Input: part model. Units: mm. Frame: model coordinates. Face numbers are marked on the shaded views. Coordinates: 2 decimals unless noted, no trailing zeros. Loops run counter-clockwise (first coordinate to the right, second up) from the corner with the lowest first, then second, coordinate; pieces in that order, holes last.
Item 1: Ray query, line 1 along Z through (x, y) = (0, 2.2); line 2 along X through (y, z) = (1.1, 0); line 3 along Z through (x, y) = (-5.5, 4.6). Return the intervals inside material, ascending.
Item 2: Pull-direction query (X, two-part tool) for the marked faces 1, 2 and 3; classes: released by +X, released by -X, zero draft, split by the parting line, or undercut.
Item 3: Contact query for flat-ended pins moving along their axis: P1, Ø6, axis at x = 4, z = 1.5, coming from the -Y side; P2, Ø2, axis at y = 2.5, z = 5.5, coming from the +X side; P3, Ø1.5, axis at x = 0, z = 0, coming from the -Y side. Output: stop coordinate, or through.
Item 4: Section B-B on x = -9.5. Return loops of the section in (y, z).
Item 5: Section C-C on z = -8. Return loops of the section in (x, y), and give its area (3 significant figures).
```python
from build123d import *

# Parameters (mm, degrees)
SKETCH1_R           = 1.218989221
BOSS_EXTRUDE6_DEPTH = 5.08


with BuildPart() as part:
    # Sketch1 → Boss-Extrude6 (new body)
    with BuildSketch(Plane(origin=(0, 0, 0), x_dir=(1, 0, 0), z_dir=(0, 1, 0))):
        with BuildLine():
            ThreePointArc((-1.519001557, -12.033660962), (0, -12.662852008), (1.519001557, -12.033660962))
            Line((1.519001557, -12.033660962), (2.038136122, -11.193432272))
            ThreePointArc((2.038136122, -11.193432272), (2.034563062, -11.204068286), (2.030934498, -11.214685493))
            Line((2.030934498, -11.214685493), (10.329167319, 2.060586649))
            ThreePointArc((10.329167319, 2.060586649), (7.892426257, 9.808202336), (-0.164422722, 8.783292397))
            ThreePointArc((-0.164422722, 8.783292397), (-8.079308366, 9.623050723), (-10.561191909, 2.060586649))
            Line((-10.561191909, 2.060586649), (-9.239218773, 0))
            Line((-9.239218773, 0), (-9.150338425, -0.138539621))
            Line((-9.150338425, -0.138539621), (-2.013925132, -11.262213432))
            Line((-2.013925132, -11.262213432), (-1.519001557, -12.033660962))
        make_face()
        Circle(SKETCH1_R, mode=Mode.SUBTRACT)
    extrude(amount=BOSS_EXTRUDE6_DEPTH)


solid = part.part
```
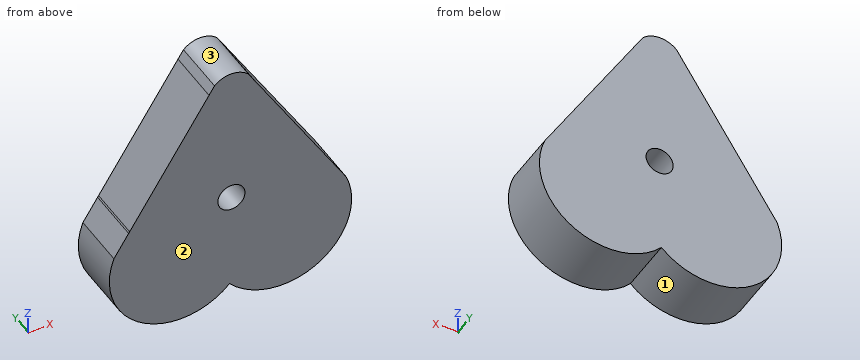
Results found:
1. line 1: z = -8.95 to -1.22, 1.22 to 12.66
1. line 2: x = -9.24 to -1.22, 1.22 to 9.04
1. line 3: z = -10.58 to 5.83
2. face 1: undercut
2. face 2: zero draft
2. face 3: split by the parting line
3. P1: stops at y = 0
3. P2: stops at x = 6.23
3. P3: passes through
4. outline: (0, -8.37) - (5.08, -8.37) - (5.08, -0.41) - (0, -0.41) - close
5. outline: (-9.78, 0) - (9.74, 0) - (9.74, 5.08) - (-9.78, 5.08) - close
5. area: 99.2 mm2
